```python
from build123d import *

# Parameters (mm, degrees)
CROQUIS2_R              = 47.5
CROQUIS2_R_2            = 15
SALIENTE_EXTRUIR1_DEPTH = 5
CORTAR_EXTRUIR1_START   = -5
CORTAR_EXTRUIR1_DEPTH   = 5
SALIENTE_EXTRUIR2_DEPTH = 35


with BuildPart() as part:
    # Croquis2 → Saliente-Extruir1 (new body)
    with BuildSketch(Plane(origin=(0, 40, 0), x_dir=(1, 0, 0), z_dir=(0, 1, 0))):
        with Locations(Location((0, 0, 0), (0, 0, 270))):
            Circle(CROQUIS2_R)
        with Locations(Location((0, 0, 0), (0, 0, 270))):
            Circle(CROQUIS2_R_2, mode=Mode.SUBTRACT)
    extrude(amount=-SALIENTE_EXTRUIR1_DEPTH)

    # Croquis3 → Cortar-Extruir1 (cut)
    with BuildSketch(Plane.XZ.offset(-35).offset(CORTAR_EXTRUIR1_START)):
        with BuildLine():
            Line((-11.990224978, 41.814883773), (-13.092774401, 45.659930557))
            ThreePointArc((-13.092774401, 45.659930557), (0, 47.5), (13.092774401, 45.659930557))
            Line((13.092774401, 45.659930557), (11.990224978, 41.814883773))
            ThreePointArc((11.990224978, 41.814883773), (0, 43.5), (-11.990224978, 41.814883773))
        make_face()
        with BuildLine():
            Line((30.217639115, -31.291281315), (32.996272597, -34.168640516))
            ThreePointArc((32.996272597, -34.168640516), (41.13620668, -23.75), (46.089046998, -11.491290041))
            Line((46.089046998, -11.491290041), (42.207864093, -10.523602459))
            ThreePointArc((42.207864093, -10.523602459), (37.672105065, -21.75), (30.217639115, -31.291281315))
        make_face()
        with BuildLine():
            Line((-42.207864093, -10.523602459), (-46.089046998, -11.491290041))
            ThreePointArc((-46.089046998, -11.491290041), (-41.13620668, -23.75), (-32.996272597, -34.168640516))
            Line((-32.996272597, -34.168640516), (-30.217639115, -31.291281315))
            ThreePointArc((-30.217639115, -31.291281315), (-37.672105065, -21.75), (-42.207864093, -10.523602459))
        make_face()
    extrude(amount=CORTAR_EXTRUIR1_DEPTH, mode=Mode.SUBTRACT)

    # Croquis4 → Saliente-Extruir2 (add)
    with BuildSketch(Plane.XZ.offset(-35)):
        with BuildLine():
            Line((-43.493374739, 0.75917968), (-47.49276552, 0.828989306))
            ThreePointArc((-47.49276552, 0.828989306), (-47.194663145, -5.377152654), (-46.089046998, -11.491290041))
            Line((-46.089046998, -11.491290041), (-42.207864093, -10.523602459))
            ThreePointArc((-42.207864093, -10.523602459), (-43.220375722, -4.924339799), (-43.493374739, 0.75917968))
        make_face()
        with BuildLine():
            Line((-22.404156259, 37.286777581), (-24.464308558, 40.715446783))
            ThreePointArc((-24.464308558, 40.715446783), (-18.940580774, 43.560353533), (-13.092774401, 45.659930557))
            Line((-13.092774401, 45.659930557), (-11.990224978, 41.814883773))
            ThreePointArc((-11.990224978, 41.814883773), (-17.345584498, 39.892113236), (-22.404156259, 37.286777581))
        make_face()
        with BuildLine():
            Line((43.493374739, 0.75917968), (47.49276552, 0.828989306))
            ThreePointArc((47.49276552, 0.828989306), (47.194663145, -5.377152654), (46.089046998, -11.491290041))
            Line((46.089046998, -11.491290041), (42.207864093, -10.523602459))
            ThreePointArc((42.207864093, -10.523602459), (43.220375722, -4.924339799), (43.493374739, 0.75917968))
        make_face()
        with BuildLine():
            Line((22.404156259, 37.286777581), (24.464308558, 40.715446783))
            ThreePointArc((24.464308558, 40.715446783), (18.940580774, 43.560353533), (13.092774401, 45.659930557))
            Line((13.092774401, 45.659930557), (11.990224978, 41.814883773))
            ThreePointArc((11.990224978, 41.814883773), (17.345584498, 39.892113236), (22.404156259, 37.286777581))
        make_face()
        with BuildLine():
            Line((-21.089218481, -38.045957261), (-23.028456962, -41.544436089))
            ThreePointArc((-23.028456962, -41.544436089), (-28.254082371, -38.183200879), (-32.996272597, -34.168640516))
            Line((-32.996272597, -34.168640516), (-30.217639115, -31.291281315))
            ThreePointArc((-30.217639115, -31.291281315), (-25.874791224, -34.967773437), (-21.089218481, -38.045957261))
        make_face()
        with BuildLine():
            Line((21.089218481, -38.045957261), (23.028456962, -41.544436089))
            ThreePointArc((23.028456962, -41.544436089), (28.254082371, -38.183200879), (32.996272597, -34.168640516))
            Line((32.996272597, -34.168640516), (30.217639115, -31.291281315))
            ThreePointArc((30.217639115, -31.291281315), (25.874791224, -34.967773437), (21.089218481, -38.045957261))
        make_face()
    extrude(amount=SALIENTE_EXTRUIR2_DEPTH)


solid = part.part
```
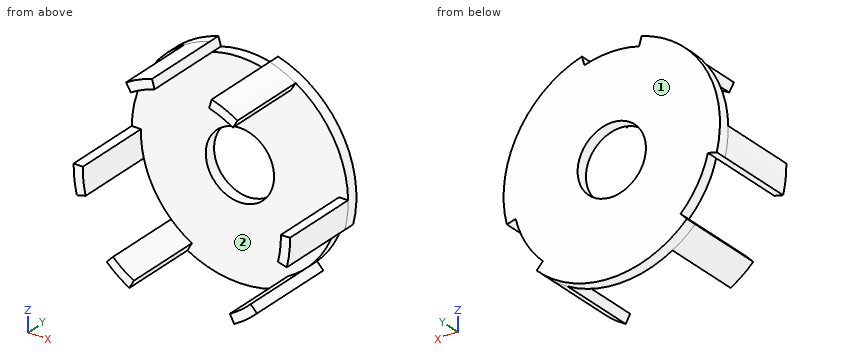
Check sheet for the modelled part. Datum: model origin and axes. Units: mm. Face numbers are marked on the shaded views. Round coordinates to 2 decimals unless told otherwise and drop trailing zeros. Loops run counter-clockwise (first coordinate to the right, second up) from the corner with the lowest first, then second, coordinate; pieces in that order, holes last. Notation, with made-up numbers: (40.5, 88) - (98.5, 88) arc R29 cw to (98.5, 108) - close; hole circle Ø8 at (-25, 15.25). An arc over 180 degrees is marked (long way). Write item = value, one per line. Start each with the question number.
Q1. Section check D-D (z = -8). Record the boundary of the cut face in (x, y).
Q2. Depth check by flat-ended pin: P1, Ø1.5, axis at x = -24.5, y = 19, coming from the +Z side; P2, Ø6, axis at x = 25.5, y = 10, coming from the -Z side; P3, Ø18, axis at x = 0, z = 0, coming from the +Y side; P4, Ø2, axis at x = -13.5, z = -17.5, coming from the -Y side. Enter the tip coordinate at first touch or a pass-through.
Q3. Section check B-B (y = 16). Record the boundary of the cut face in (x, z).
Q4. Thickness scan on L1, parallel to X at y = 36.75, z = 0; L2, parallel to Y at x = 5, z = -29.5; L3, parallel to X at y = 37, z = -8. Record the ranges inside material, lowest first.
Q5. Section check A-A (x = 0). Record the boundary of the cut face in (y, z), plus the area to 3 significant figures.
Q6. Release check for a two-part mould opening along Z. For the marked faces 1 and 2 record: pulls with the +Z half, pulls with the -Z half, needs draft (parallel to the pull), parting line crosses it, or undercut.
Q7. Section check C-C (z = 7). Record the boundary of the cut face in (x, y), plus the area to 3 significant figures.
Derived:
q1.outline = (-46.82, 0) - (-42.76, 0) - (-42.76, 35) - (-12.69, 35) - (-12.69, 40) - (-46.82, 40) - close; (12.69, 35) - (42.76, 35) - (42.76, 0) - (46.82, 0) - (46.82, 40) - (12.69, 40) - close
q2.P1 = 41.14
q2.P2 = -41.54
q2.P3 = through
q2.P4 = 35
q3.outline = (-47.49, 0.83) arc R47.5 ccw to (-46.09, -11.49) - (-42.21, -10.52) arc R43.5 cw to (-43.49, 0.76) - close; (-33, -34.17) arc R47.5 ccw to (-23.03, -41.54) - (-21.09, -38.05) arc R43.5 cw to (-30.22, -31.29) - close; (-24.46, 40.72) - (-22.4, 37.29) arc R43.5 cw to (-11.99, 41.81) - (-13.09, 45.66) arc R47.5 ccw to start; (11.99, 41.81) arc R43.5 cw to (22.4, 37.29) - (24.46, 40.72) arc R47.5 ccw to (13.09, 45.66) - close; (21.09, -38.05) - (23.03, -41.54) arc R47.5 ccw to (33, -34.17) - (30.22, -31.29) arc R43.5 cw to start; (42.21, -10.52) - (46.09, -11.49) arc R47.5 ccw to (47.49, 0.83) - (43.49, 0.76) arc R43.5 cw to start
q4.L1 = -47.5 to -15, 15 to 47.5
q4.L2 = 35 to 40
q4.L3 = -46.82 to -12.69, 12.69 to 46.82
q5.outline = (35, -47.5) - (40, -47.5) - (40, -15) - (35, -15) - close; (35, 15) - (40, 15) - (40, 43.5) - (35, 43.5) - close
q5.area = 305 mm^2
q6.face_1 = needs draft
q6.face_2 = undercut
q7.outline = (-46.98, 35) - (-13.27, 35) - (-13.27, 40) - (-46.98, 40) - close; (13.27, 35) - (46.98, 35) - (46.98, 40) - (13.27, 40) - close
q7.area = 337 mm^2
